Answer from the drawing. Dimensions are ordinates in mm from the lowest x, y and z of the part. Round coordinates to 2 decimals unless told otherwise and drop trailing zeros. Loops run counter-clockwise (first coordinate to the right, second up) from the corner with the lowest first, then second, coordinate; pieces in that order, holes last. Notation, with made-up numbers: (89, 70.5) - (119, 70.5) arc R21 ccw to (119, 88.5) - close; hole circle Ø3 at (-4.75, 53.5). An arc over 180 degrees is marked (long way). Answer as CSV lines item,"result".
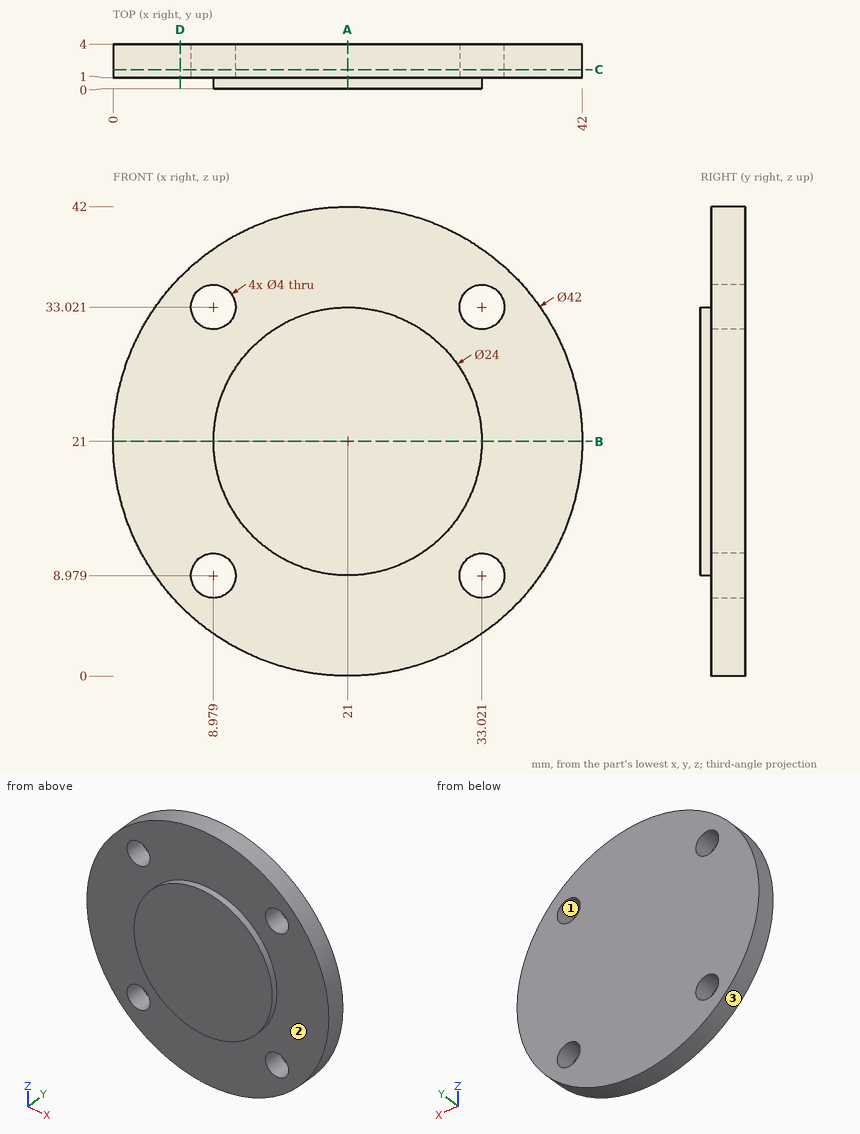
1) A cutting plane is placed at D-D, the plane x = 6. Determine the outline of the cut face in (y, z).
Entries:
outline,"(1, 6.3) - (4, 6.3) - (4, 35.7) - (1, 35.7) - close"
2) Each of these flat-tipped pins is pushed along its axis until it touches: P1, Ø1, axis at y = 3.5, z = 22.5, coming from the +X side; P2, Ø1, axis at y = 1, z = 31.5, coming from the +X side; P3, Ø2, axis at x = 20, y = 0.5, coming from the -Z side. Where does it stop, or does it pass through?
Entries:
P1,"stops at x = 41.98"
P2,"stops at x = 39.47"
P3,"stops at z = 0"
3) Find the intervals of material crossed by line 1 (X direction, y = 1.55, z = 34) (1 decimal); line 2 (Z direction, x = 21.5, y = 1.7); line 3 (Y direction, x = 4, z = 20), in increasing order.
Entries:
line 1,"x = 4.5 to 7.2, 10.7 to 31.3, 34.8 to 37.5"
line 2,"z = 0.01 to 41.99"
line 3,"y = 1 to 4"
4) The mould has two halves that part along Z. Classify the marked faces 1, 2 and 3: pulls with the +Z half, pulls with the -Z half, needs draft (parallel to the pull), parting line crosses it, or undercut.
Entries:
face 1,"undercut"
face 2,"needs draft"
face 3,"parting line crosses it"
5) A cutting plane is placed at A-A, the plane x = 21. Determine the outline of the cut face in (y, z), plus the area to 3 significant figures.
Entries:
outline,"(0, 9) - (1, 9) - (1, 0) - (4, 0) - (4, 42) - (1, 42) - (1, 33) - (0, 33) - close"
area,"150 mm^2"
6) A cutting plane is placed at B-B, the plane z = 21. Determine the outline of the cut face in (x, y).
Entries:
outline,"(0, 1) - (9, 1) - (9, 0) - (33, 0) - (33, 1) - (42, 1) - (42, 4) - (0, 4) - close"
7) A cutting plane is placed at C-C, the plane y = 1.7. Determine the outline of the cut face in (x, z), plus the area to 3 significant figures.
Entries:
outline,"circle Ø42 at (21, 21); hole circle Ø4 at (8.98, 8.98); hole circle Ø4 at (8.98, 33.02); hole circle Ø4 at (33.02, 8.98); hole circle Ø4 at (33.02, 33.02)"
area,"1,340 mm^2"
